Part model, mm, in its own coordinate system. A direction names the side the tool comes from. Coordinates: 2 decimals unless noted, no trailing zeros. Order: outer loops, then holes, each group sorted by start corner. A loop starts at its lowest first (then second) coordinate and runs counter-clockwise, first axis right, second up.
from build123d import *

# Parameters (mm, degrees)
F1_DEPTH  = 40
F4_DEPTH  = 10
F6_DEPTH  = 20
F8_DEPTH  = 5
F10_DEPTH = 5


with BuildPart() as f1:
    # F0 (on Top) → F1 (new body)
    with BuildSketch(Plane.XY):
        Polygon((20, 11.547005), (-20, 11.547005), (0, -23.094011), align=None)
    extrude(amount=F1_DEPTH)

    # F3 (on face) → F4 (cut)
    with BuildSketch(Plane.XY.offset(40)):
        Polygon((0, -23.094011), (6.666667, 11.547005), (-20, 11.547005), align=None)
    extrude(amount=-F4_DEPTH, mode=Mode.SUBTRACT)

    # F5 (on face) → F6 (cut)
    with BuildSketch(Plane.XY.offset(40)):
        Polygon((0, -23.094011), (-6.666667, 11.547005), (-20, 11.547005), align=None)
    extrude(amount=-F6_DEPTH, mode=Mode.SUBTRACT)

    # F7 (on face) → F8 (join)
    with BuildSketch(Plane.XY.offset(30)):
        Polygon((0, 11.547005), (0, -23.094011), (6.666667, 11.547005), align=None)
    extrude(amount=F8_DEPTH)

    # F9 (on face) → F10 (join)
    with BuildSketch(Plane.XY.offset(20)):
        Polygon((-6.666667, 11.547005), (-13.333333, 11.547005), (0, -23.094011), align=None)
    extrude(amount=F10_DEPTH)


solid = f1.part
Q1. Which spindle directions (+Z, -Z, +X, -X, +Y, -Y) get a long thin tool onto all of the face, cutting with end or side? Do faces 1 (the face through (-7, 1, 25)), 2 (the face through (0, -6, 32)), 3 (the face through (10, -2, 40)), 4 (the face through (3.287, -6.016, 37.535)), 5 (the face through (-10.14, -5.53, 9.86)). Say none if no direction does.
Results list:
face 1: +Z, -X, -Y
face 2: +Z, -X, +Y, -Y
face 3: +Z, +X, -X, +Y, -Y
face 4: +Z, -X, +Y
face 5: +Z, -Z, -X, -Y
Q2. Cut at A-A on y = -12. Write the cut outline in (x, z), and give its area (3 significant figures).
Results list:
outline: (-6.41, 0) - (6.41, 0) - (6.41, 40) - (2.14, 40) - (2.14, 35) - (0, 35) - (0, 30) - (-2.14, 30) - (-2.14, 25) - (-4.27, 25) - (-4.27, 20) - (-6.41, 20) - close
area: 406 mm2
Q3. Pin check, flat tips, straight feed: pin 1 Ø3.5 at (x, y) = (-3.5, -9.5) entering from +Z; pin 2 Ø1 at (y, z) = (3.5, 31.5) entering from +X; pin 3 Ø1 at (x, z) = (3.5, 29) entering from -Y. Stop position of each tip, or through.
Results list:
pin 1: stops at z = 30
pin 2: stops at x = 15.64
pin 3: stops at y = -17.9
Q4. Cut at D-D on y = 0.5. Write the cut outline in (x, z).
Results list:
outline: (-13.62, 0) - (13.62, 0) - (13.62, 40) - (4.54, 40) - (4.54, 35) - (0, 35) - (0, 30) - (-4.54, 30) - (-4.54, 25) - (-9.08, 25) - (-9.08, 20) - (-13.62, 20) - close
Q5. Cut at C-C on x = 5.5. Write the cut outline in (y, z), and give its area (3 significant figures).
Results list:
outline: (-13.57, 0) - (11.55, 0) - (11.55, 35) - (5.48, 35) - (5.48, 40) - (-13.57, 40) - close
area: 974 mm2
Q6. Cut at B-B on z = 36.5. Write the cut outline in (x, y), and give its area (3 significant figures).
Results list:
outline: (0, -23.09) - (20, 11.55) - (6.67, 11.55) - close
area: 231 mm2
Q7. Wall check: line 1 along Z through (x, y) = (-4.5, 4); line 2 along Z through (x, y) = (-6, -10); line 3 along Y through (x, z) = (0.5, 14). Give the ranges that are in metal, low to high.
Results list:
line 1: z = 0 to 30
line 2: z = 0 to 20
line 3: y = -22.23 to 11.55
